Geometry: see drawing. Coordinates: mm, zero at the bounding-box minimum. A direction names the side the tool comes from. Round coordinates to 2 decimals unless told otherwise and drop trailing zeros. Order: outer loops, then holes, each group sorted by start corner. A loop starts at its lowest first (then second) coordinate and runs counter-clockwise, first axis right, second up. Notation, with made-up numbers: (46, 7) -> (70, 7) arc R24 ccw to (70, 45) -> close; hole circle Ø9 at (81.25, 80.25). An arc over 180 degrees is marked (long way). Answer as CSV lines item,"result". Start each with the question number.
(1) Section query A-A (z = 15). Output: boundary loops of the cut face in (x, y), plus the area to 3 significant figures.
(2) Section query B-B (x = 22). Output: boundary loops of the cut face in (y, z), plus the area to 3 significant figures.
(3) Line query: line 1 along X through (y, z) = (11.75, 23); line 2 along Y through (x, z) = (13, 23.5). Output: solid intervals per line, ascending. Write a range as from..to.
(4) Contact query for flat-ended pins moving along their axis: P1, Ø12, axis at x = 7.5, y = 13.5, coming from the -Z side; P2, Ø13.5, axis at x = 35.5, z = 20.5, coming from the -Y side; P3, Ø6, axis at y = 6, z = 37, coming from the +X side; P4, Ø10, axis at y = 13, z = 42.5, coming from the -X side. Output: stop coordinate, or through.
(5) Set-up query: the marked faces 1, 2 and 3. Return all of +Z, -Z, +X, -X, +Y, -Y with unobstructed straight access to the full face (end or side cutting, diameter ignored); none if empty.
(6) Section query D-D (x = 26). Output: boundary loops of the cut face in (y, z).
(7) Section query C-C (z = 6). Output: boundary loops of the cut face in (x, y).
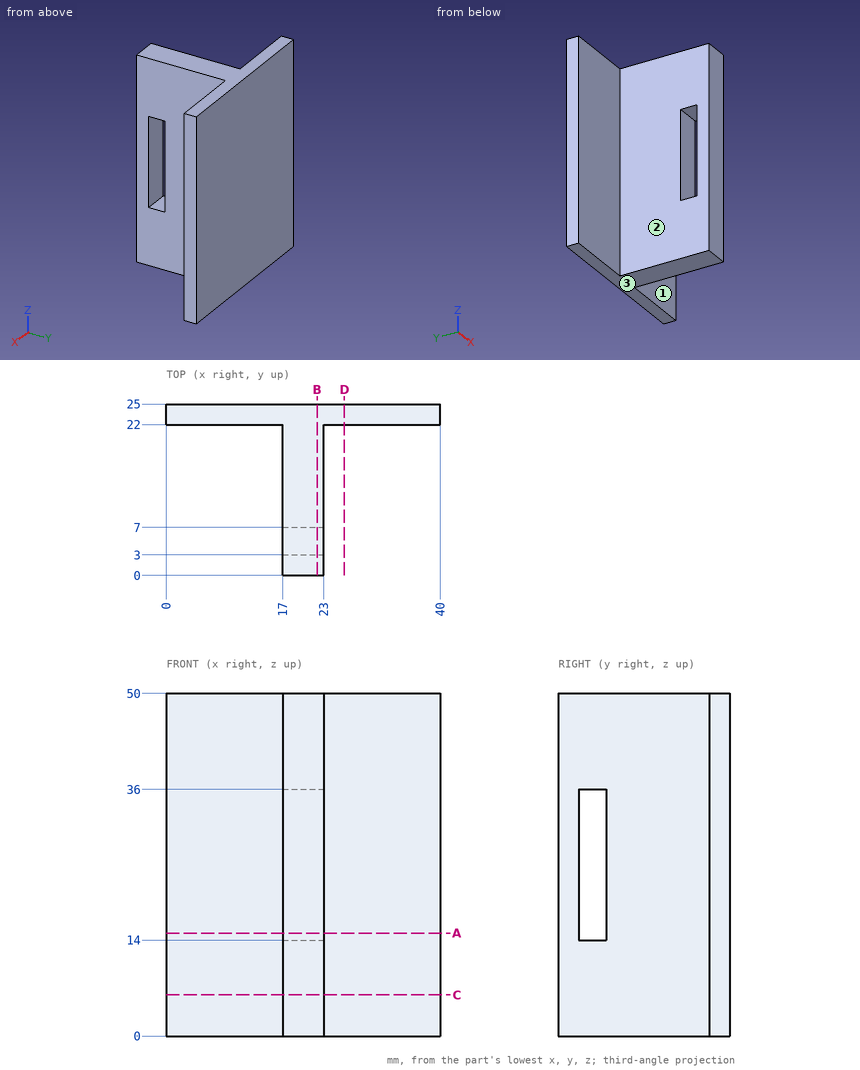
Answer block:
1,outline,"(0, 22) -> (17, 22) -> (17, 7) -> (23, 7) -> (23, 22) -> (40, 22) -> (40, 25) -> (0, 25) -> close; (17, 0) -> (23, 0) -> (23, 3) -> (17, 3) -> close"
1,area,"228 mm2"
2,outline,"(0, 0) -> (25, 0) -> (25, 50) -> (0, 50) -> close; hole (3, 14) -> (7, 14) -> (7, 36) -> (3, 36) -> close"
2,area,"1,160 mm2"
3,line 1,"17..23"
3,line 2,"22..25"
4,P1,"through"
4,P2,"y = 22"
4,P3,"x = 23"
4,P4,"x = 17"
5,face 1,"+Z, -Z, +X, -Y"
5,face 2,"+Z, -Z, -X, -Y"
5,face 3,"-Z, +X, -X, +Y, -Y"
6,outline,"(22, 0) -> (25, 0) -> (25, 50) -> (22, 50) -> close"
7,outline,"(0, 22) -> (17, 22) -> (17, 0) -> (23, 0) -> (23, 22) -> (40, 22) -> (40, 25) -> (0, 25) -> close"
